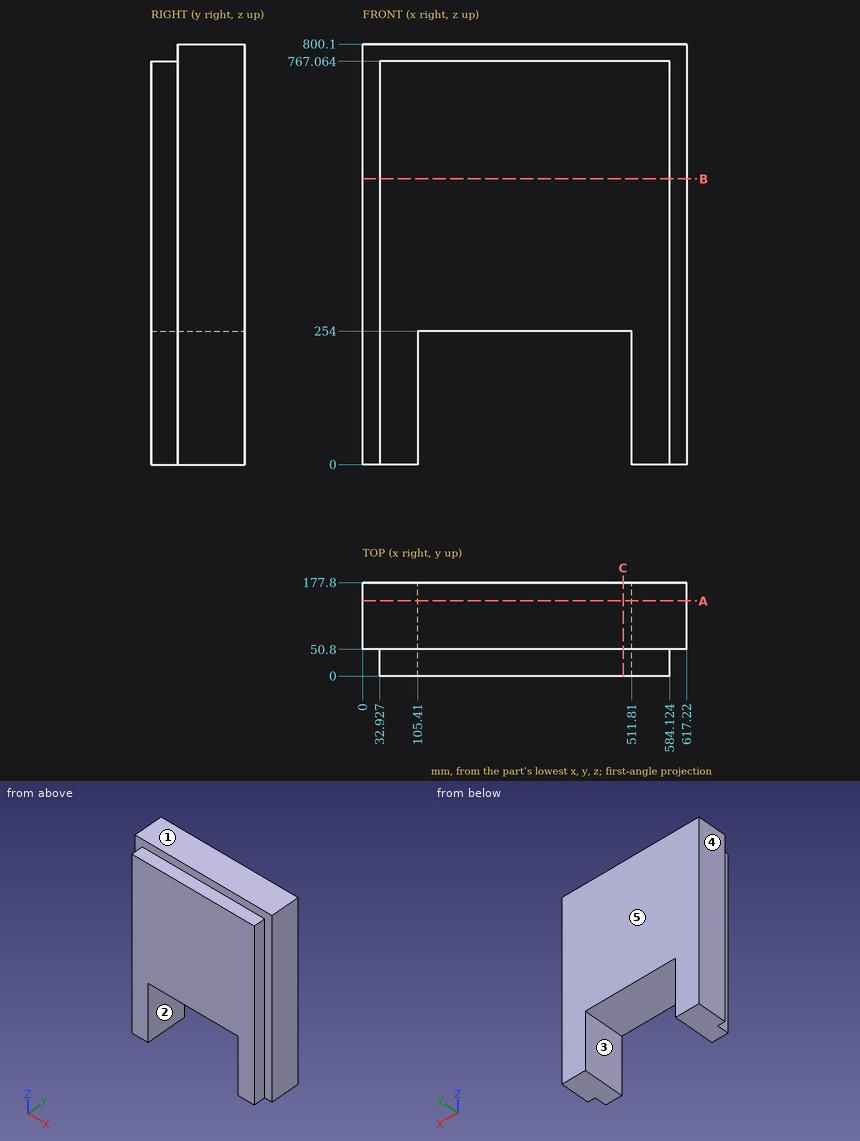
Check sheet for the drawn part. Datum: minimum x, y, z corner. Units: mm. A direction names the side the tool comes from. Round coordinates to 2 decimals unless told otherwise and drop trailing zeros. Order: outer loops, then holes, each group sorted by start corner. A loop starts at its lowest first (then second) coordinate and runs counter-clockwise, first axis right, second up.
1) Mould release check, pull along X, two halves, no side actions. Record for the marked faces 3, 4 and 5: +X half, -X half, draft (parallel to the pull), parting line (faces both ways), or undercut.
2) Go/stop test with flat-tipped pins: pin 1 Ø10 at (y, z) = (27.5, 684) entering from +X; pin 2 Ø15 at (y, z) = (36.5, 515.5) entering from -X; pin 3 Ø6 at (x, y) = (183, 59) entering from -Z. Record where each tip stops, or that it passes through.
3) Section check C-C (x = 496). Record the boundary of the cut face in (y, z).
4) Section check A-A (y = 143). Record the boundary of the cut face in (x, z).
5) Scan lines: line 1 (X direction, y = 169.5, z = 216); line 2 (X direction, y = 21, z = 75.5); line 3 (Z direction, x = 429.5, y = 87.5). Record each from-to range of solid material in increasing order.
6) Section check B-B (z = 543.5). Record the boundary of the cut face in (x, y), and give its area (3 significant figures).
7) Tool access check on the marked faces 1 and 2. Record the directions out of +Z, -Z, +X, -X, +Y, -Y that give a thin tool (end or side, any length) a straight path to the whole face; none if there is none.
Result:
1. face 3: undercut
1. face 4: -X half
1. face 5: draft
2. pin 1: stops at x = 584.12
2. pin 2: stops at x = 32.93
2. pin 3: stops at z = 254
3. outline: (0, 254) - (177.8, 254) - (177.8, 800.1) - (50.8, 800.1) - (50.8, 767.06) - (0, 767.06) - close
4. outline: (0, 0) - (105.41, 0) - (105.41, 254) - (511.81, 254) - (511.81, 0) - (617.22, 0) - (617.22, 800.1) - (0, 800.1) - close
5. line 1: x = 0 to 105.41, 511.81 to 617.22
5. line 2: x = 32.93 to 105.41, 511.81 to 584.12
5. line 3: z = 254 to 800.1
6. outline: (0, 50.8) - (32.93, 50.8) - (32.93, 0) - (584.12, 0) - (584.12, 50.8) - (617.22, 50.8) - (617.22, 177.8) - (0, 177.8) - close
6. area: 106,000 mm2
7. face 1: +Z, +X, -X, +Y, -Y
7. face 2: -Z, +Y, -Y
